For this review, take the finished solid that the model builds, in its own axes (mm). A direction names the side the tool comes from. Round coordinates to 2 decimals unless told otherwise and drop trailing zeros. Order: outer loops, then holes, each group sorted by start corner. A loop starts at its lowest first (then second) coordinate and runs counter-clockwise, first axis right, second up. Notation, with made-up numbers: (14.5, 12) - (47.5, 12) arc R8 cw to (47.5, 19) - close; hole circle Ø3 at (57, 62). An arc over 180 degrees is marked (long way). One line per question, with ' | ' between items.
Autodesk Inventor part; units mm, degrees
ref_plane "YZ Plane" through (0, 0, 0) normal (1, 0, 0) x (0, 1, 0)
ref_plane "XZ Plane" through (0, 0, 0) normal (0, 1, 0) x (-1, 0, 0)
ref_plane "XY Plane" through (0, 0, 0) normal (0, 0, 1) x (1, 0, 0)
sketch "Sketch1" plane through (0, 0, 0) normal (0, 0, 1) x (1, 0, 0)
  line L0 (0, 0) -> (41.5, 0)
  line L1 (41.5, 0) -> (41.5, -73)
  line L2 (41.5, -73) -> (0, -73)
  line L3 (0, -73) -> (0, 0)
  line L4 (0, -73) -> (3.11, -73)
  line L5 (0, -73) -> (3.11, -73) construction
  line L6 (3.11, -73) -> (3.11, -69.85)
  line L7 (3.11, -73) -> (6.26, -73) construction
  line L8 (3.11, -69.85) -> (14.54, -69.85)
  line L9 (14.54, -69.85) -> (19.65, -69.85)
  line L10 (19.65, -69.85) -> (31.08, -69.85)
  circle A0 centre (3.11, -69.85) radius 1.6
  circle A1 centre (14.54, -69.85) radius 1.6
  circle A2 centre (19.65, -69.85) radius 1.6
  circle A3 centre (31.08, -69.85) radius 1.6
  line L11 (3.11, -69.85) -> (3.11, -55.42)
  line L12 (3.11, -69.85) -> (17.54, -69.85) construction
  line L13 (0, -73) -> (4.33, -73)
  line L14 (0, -73) -> (4.33, -73) construction
  line L15 (4.33, -73) -> (4.33, -53.49)
  line L16 (3.11, -55.42) -> (6.6479, -55.42)
  circle A4 centre (4.33, -55.42) radius 1.651
  line L17 (4.33, -55.42) -> (4.33, -37.69)
  line L18 (4.33, -55.42) -> (22.06, -55.42) construction
  line L19 (4.33, -55.42) -> (29.68, -55.42)
  line L20 (4.33, -55.42) -> (29.68, -55.42) construction
  circle A5 centre (4.33, -37.69) radius 1.651
  circle A6 centre (29.68, -55.42) radius 1.651
  line L21 (4.33, -37.69) -> (39.0376, -37.69)
  line L22 (29.68, -55.42) -> (29.68, -25.3245)
  circle A7 centre (29.68, -37.69) radius 1.651
  line L23 (4.33, -37.69) -> (4.33, -30.44)
  line L24 (4.33, -37.69) -> (11.58, -37.69) construction
  line L25 (4.33, -30.44) -> (4.33, -12.71)
  line L26 (4.33, -30.44) -> (29.68, -30.44)
  line L27 (4.33, -30.44) -> (29.68, -30.44) construction
  line L28 (4.33, -12.71) -> (29.68, -12.71)
  circle A8 centre (29.48, -12.71) radius 1.651
  circle A9 centre (4.33, -12.71) radius 1.651
  circle A10 centre (4.33, -30.44) radius 1.651
  circle A11 centre (29.68, -30.44) radius 1.651
  dimension "d0" = 41.5
  dimension "d1" = 73
  dimension "d2" = 3.11
  dimension "d3" = 0
  dimension "d4" = 3.15
  dimension "d5" = 90
  dimension "d6" = 11.43
  dimension "d7" = 90
  dimension "d9" = 5.11
  dimension "d10" = 11.43
  dimension "d11" = 180
  dimension "d12" = 3.2
  dimension "d13" = 3.2
  dimension "d14" = 3.2
  dimension "d15" = 3.2
  dimension "d18" = 14.43
  dimension "d19" = 90
  dimension "d20" = 4.33
  dimension "d21" = 0
  dimension "d22" = 3.302
  dimension "d23" = 17.73
  dimension "d24" = 90
  dimension "d25" = 25.35
  dimension "d26" = 0
  dimension "d27" = 3.302
  dimension "d28" = 3.302
  dimension "d29" = 3.302
  dimension "d30" = 7.25
  dimension "d31" = 90
  dimension "d32" = 17.73
  dimension "d33" = 180
  dimension "d34" = 25.35
  dimension "d35" = 0
  dimension "d36" = 25.35
  dimension "d37" = 3.302
  dimension "d38" = 3.302
  dimension "d39" = 3.302
  dimension "d40" = 3.302
extrude "Extrusion2" add sketch "Sketch1" along normal blind 4 contours L0 L1 L2 L15 A0 A4 L16 L19 A6 L22 A7 A11 L26 A10 L23 A5 L17 L11 L6 L3 | L6 A0 L15 L2 | L11 A4 L15 A0 | L15 L17 A5 L21 A7 L22 A6 L19 L16 A4 | L23 A10 L26 A11 L22 A7 L21 A5
sketch "Sketch3" plane through (0, 0, 4) normal (0, 0, 1) x (1, 0, 0)
  circle A0 centre (4.33, -55.42) radius 1.651
  circle A1 centre (4.33, -55.42) radius 3.5
  circle A2 centre (29.68, -55.42) radius 1.651
  circle A3 centre (29.68, -55.42) radius 3.5
  circle A4 centre (4.33, -12.71) radius 1.651
  circle A5 centre (4.33, -12.71) radius 3.5
  circle A6 centre (29.48, -12.71) radius 1.651
  circle A7 centre (29.48, -12.71) radius 3.5
  point P0 (0, 0)
  dimension "d46" = 7
  dimension "d47" = 7
  dimension "d48" = 7
  dimension "d49" = 7
extrude "Extrusion4" add sketch "Sketch3" along normal blind 15
sketch "Sketch8" plane through (0, 0, 0) normal (0, 0, -1) x (-1, 0, 0)
  circle A0 centre (-4.33, -12.71) radius 1.651
  circle A1 centre (-4.33, -12.71) radius 3
  circle A2 centre (-29.48, -12.71) radius 1.651
  circle A3 centre (-29.48, -12.71) radius 3
  circle A4 centre (-29.68, -55.42) radius 1.651
  circle A5 centre (-29.68, -55.42) radius 3
  circle A6 centre (-4.33, -55.42) radius 1.651
  circle A7 centre (-4.33, -55.42) radius 3
  line L0 (-1.33, -12.71) -> (-2.83, -15.3081)
  line L1 (-2.83, -15.3081) -> (-5.83, -15.3081)
  line L2 (-5.83, -15.3081) -> (-7.33, -12.71)
  line L3 (-7.33, -12.71) -> (-5.83, -10.1119)
  line L4 (-5.83, -10.1119) -> (-2.83, -10.1119)
  line L5 (-2.83, -10.1119) -> (-1.33, -12.71)
  circle A8 centre (-29.48, -12.71) radius 3.5
  line L6 (-25.98, -12.71) -> (-27.73, -15.7411)
  line L7 (-27.73, -15.7411) -> (-31.23, -15.7411)
  line L8 (-31.23, -15.7411) -> (-32.98, -12.71)
  line L9 (-32.98, -12.71) -> (-31.23, -9.6789)
  line L10 (-31.23, -9.6789) -> (-27.73, -9.6789)
  line L11 (-27.73, -9.6789) -> (-25.98, -12.71)
  line L12 (-26.68, -55.42) -> (-28.18, -58.0181)
  line L13 (-28.18, -58.0181) -> (-31.18, -58.0181)
  line L14 (-31.18, -58.0181) -> (-32.68, -55.42)
  line L15 (-32.68, -55.42) -> (-31.18, -52.8219)
  line L16 (-31.18, -52.8219) -> (-28.18, -52.8219)
  line L17 (-28.18, -52.8219) -> (-26.68, -55.42)
  line L18 (-1.33, -55.405) -> (-2.817, -58.0105)
  line L19 (-2.817, -58.0105) -> (-5.817, -58.0256)
  line L20 (-5.817, -58.0256) -> (-7.33, -55.435)
  line L21 (-7.33, -55.435) -> (-5.843, -52.8295)
  line L22 (-5.843, -52.8295) -> (-2.843, -52.8144)
  line L23 (-2.843, -52.8144) -> (-1.33, -55.405)
  point P0 (0, 0)
  dimension "d53" = 6
  dimension "d55" = 6
  dimension "d56" = 6
  dimension "d54" = 6
extrude "Extrusion5" cut sketch "Sketch8" against normal blind 2 contours L0 L1 L2 L3 L4 L5 | A2 | A3 | L12 L13 L14 L15 L16 L17 | L18 L19 L20 L21 L22 L23 | L6 L7 L8 L9 L10 L11
sketch "Sketch9" plane through (0, 0, 4) normal (0, 0, 1) x (1, 0, 0)
  circle A0 centre (4.33, -30.44) radius 1.651
  circle A1 centre (4.33, -30.44) radius 1.651
  circle A2 centre (4.33, -37.69) radius 1.651
  circle A3 centre (4.33, -37.69) radius 1.651
  line L0 (7.33, -30.44) -> (5.83, -33.0381)
  line L1 (5.83, -33.0381) -> (2.83, -33.0381)
  line L2 (2.83, -33.0381) -> (1.33, -30.44)
  line L3 (1.33, -30.44) -> (2.83, -27.8419)
  line L4 (2.83, -27.8419) -> (5.83, -27.8419)
  line L5 (5.83, -27.8419) -> (7.33, -30.44)
  line L6 (7.33, -37.69) -> (5.83, -40.2881)
  line L7 (5.83, -40.2881) -> (2.83, -40.2881)
  line L8 (2.83, -40.2881) -> (1.33, -37.69)
  line L9 (1.33, -37.69) -> (2.83, -35.0919)
  line L10 (2.83, -35.0919) -> (5.83, -35.0919)
  line L11 (5.83, -35.0919) -> (7.33, -37.69)
  line L12 (8.33, -30.44) -> (6.33, -33.9041)
  line L13 (6.33, -33.9041) -> (2.33, -33.9041)
  line L14 (2.33, -33.9041) -> (0.33, -30.44)
  line L15 (0.33, -30.44) -> (2.33, -26.9759)
  line L16 (2.33, -26.9759) -> (6.33, -26.9759)
  line L17 (6.33, -26.9759) -> (8.33, -30.44)
  line L18 (8.33, -37.69) -> (6.33, -41.1541)
  line L19 (6.33, -41.1541) -> (2.33, -41.1541)
  line L20 (2.33, -41.1541) -> (0.33, -37.69)
  line L21 (0.33, -37.69) -> (2.33, -34.2259)
  line L22 (2.33, -34.2259) -> (6.33, -34.2259)
  line L23 (6.33, -34.2259) -> (8.33, -37.69)
  line L24 (6.33, -33.9041) -> (6.33, -34.2259)
  line L25 (2.33, -33.9041) -> (2.33, -34.2259)
  point P0 (0, 0)
  dimension "d59" = 3.302
  dimension "d60" = 3.302
extrude "Extrusion6" add sketch "Sketch9" along normal blind 2 contours L12 L13 L14 L15 L16 L17 | L24 L22 L25 L13 | L23 L18 L19 L20 L21 L22
properties part number "mountMount"
(1) Insertion check: pin 1 (6 mm diameter, centred on y = -48, z = 8.5, fed in from +X); pin 2 (2.5 mm diameter, centred on x = 4.5, y = -54.5, fed in from -Z); pin 3 (1 mm diameter, centred on y = -11.5, z = 11, fed in from -X); pin 4 (1.6 mm diameter, centred on x = 5, z = 5.5, fed in from -Y). Each pin has a flat end and moves straight along its axis. Give the tip position at first contact, or say it passes through.
Output values:
pin 1: through | pin 2: z = 2 | pin 3: x = 0.9 | pin 4: y = -58.92
(2) For probe 1 along Y at (x, z) = (4.33, 15.5); probe 2 along Y at (x, z) = (4.33, 1.9); probe 3 along Y at (x, z) = (19.65, 1.45), list the stretches that pass through material, from the lowest coordinate up. Write a range as [from, to].
Output values:
probe 1: [-58.92, -57.07], [-53.77, -51.92], [-16.21, -14.36], [-11.06, -9.21] | probe 2: [-73, -70.89], [-68.81, -58.02], [-52.82, -39.34], [-36.04, -32.09], [-28.79, -15.31], [-10.11, 0] | probe 3: [-73, -71.45], [-68.25, 0]
(3) We need section B-B on y = -69.85. State the section outline as (x, z) points.
Output values:
outline: (0, 0) - (1.51, 0) - (1.51, 4) - (0, 4) - close; (4.71, 0) - (12.94, 0) - (12.94, 4) - (4.71, 4) - close; (16.14, 0) - (18.05, 0) - (18.05, 4) - (16.14, 4) - close; (21.25, 0) - (29.48, 0) - (29.48, 4) - (21.25, 4) - close; (32.68, 0) - (41.5, 0) - (41.5, 4) - (32.68, 4) - close
(4) We need section C-C on x = 19. State the section outline as (y, z) points.
Output values:
outline: (-73, 0) - (-71.31, 0) - (-71.31, 4) - (-73, 4) - close; (-68.39, 0) - (0, 0) - (0, 4) - (-68.39, 4) - close
(5) We need section A-A on z = 8.25. State the section outline as (x, y) points.
Output values:
outline: circle Ø7 at (4.33, -55.42); circle Ø7 at (4.33, -12.71); circle Ø7 at (29.48, -12.71); circle Ø7 at (29.68, -55.42); hole circle Ø3.3 at (4.33, -55.42); hole circle Ø3.3 at (4.33, -12.71); hole circle Ø3.3 at (29.48, -12.71); hole circle Ø3.3 at (29.68, -55.42)
(6) For faces 5 (the flat face through (1.344, -39.446, 4.986)), 6 (the flat face through (4, -26.976, 5)), 7 (the flat face through (30, -52.822, 1)), 8 (the flat face through (6.59, -31.72, 4.99)), 9 (the flat face through (7.344, -32.148, 4.986)), list the 3-axis set-ups (+Z, -Z, +X, -X, +Y, -Y) from which the entire face can be reached by the end or side of a thin tool; tool diameter is ignored.
Output values:
face 5: +Z, -X | face 6: +Z, +X, -X | face 7: -Z | face 8: +Z | face 9: +Z, +X
(7) Mouldability with a two-part tool opening along X and no side actions: class faces 1 (the flat face through (3, -57, 2)), 2 (the flat face through (20, 0, 2)), 3 (the flat face through (7.316, -28.684, 4.986)), 4 (the flat face through (4, -40.288, 5)) as released by +X, released by -X, zero draft, split by the parting line, or undercut.
Output values:
face 1: undercut | face 2: zero draft | face 3: released by +X | face 4: undercut
